Verification items for the finished model (mm, model axes). Face numbers are marked on the shaded views. Round coordinates to 2 decimals unless told otherwise and drop trailing zeros. Order: outer loops, then holes, each group sorted by start corner. A loop starts at its lowest first (then second) coordinate and runs counter-clockwise, first axis right, second up. Notation, with made-up numbers: M -38.5,0 L -29.5,0 A28 ccw -29.5,22 Z; hole C 5,88.25 d8. An arc over 180 degrees is marked long. Use one line per item in the form item = value. Start each with the question number.
Item 1: Cross-section at D-D on x = 14.5. Enter the section's corners in (y, z) (3 decimals).
Item 2: Cross-section at C-C on z = 0.8. Count the separate pieces of the cut face and the enclosed holes in it, then the cut area to 3 significant figures.
Item 3: Cross-section at B-B on x = -6. Enter the section's corners in (y, z) (3 decimals), then the cut area to 3 significant figures.
Item 4: Cross-section at A-A on y = -24.5. Enter the section's corners in (x, z) (3 decimals), then the cut area to 3 significant figures.
Item 5: Release check for a two-part mould opening along Z. For the marked faces 1 and 2 record: +Z half, -Z half, draft (parallel to the pull), parting line (faces both ways), or undercut.
Item 6: Go/stop test with flat-tipped pins: pin 1 Ø1.6 at (y, z) = (-81.5, 1.5) entering from +X; pin 2 Ø1.5 at (y, z) = (-7, 1.5) entering from +X; pin 3 Ø1.6 at (y, z) = (-74.5, 2) entering from -X. Record where each tip stops, or that it passes through.
Item 7: Thickness scan on probe 1 along Y at (x, z) = (-22, 1.2); probe 2 along Y at (x, z) = (-14.5, 0.75); probe 3 along X at (y, z) = (1, 1.5). Record the ranges inside material, lowest first. Write a range as [from, to].
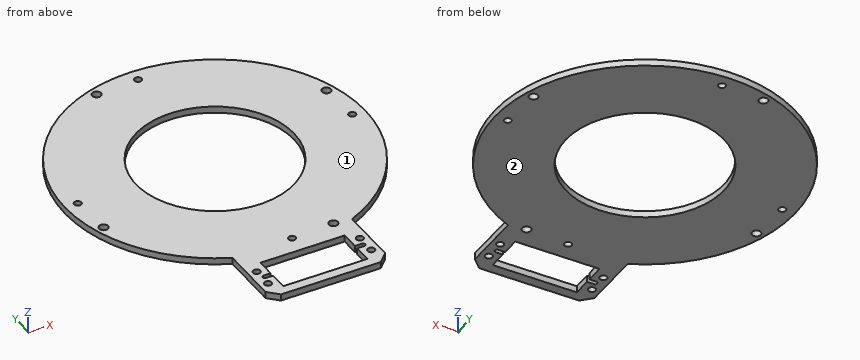
from build123d import *

# Parameters (mm, degrees)
F0_R     = 1.7272
F0_R_2   = 2.15265
F0_R_3   = 38.1
F1_DEPTH = 3.175
F2_SIZE  = 4.7625


# Not quite as in the source:
# - a feature names something its author has since deleted; it is built from what else it names


with BuildPart() as f1:
    # F0 (on Top) → F1 (new body)
    with BuildSketch(Plane.XY):
        with BuildLine():
            Line((28.86075, -99.6367724936), (28.86075, -66.3880200747))
            ThreePointArc((28.86075, -66.3880200747), (0, 72.39), (-28.86075, -66.3880200747))
            Line((-28.86075, -66.3880200747), (-28.86075, -99.6367724936))
            Line((-28.86075, -99.6367724936), (28.86075, -99.6367724936))
        make_face()
        with Locations((-24.892, -89.9847724936)):
            Circle(F0_R, mode=Mode.SUBTRACT)
        with Locations((-24.892, -80.2057724936)):
            Circle(F0_R, mode=Mode.SUBTRACT)
        with Locations((-65.2747423649, -20.5103744665)):
            Circle(F0_R_2, mode=Mode.SUBTRACT)
        with BuildLine():
            Line((-20.32, -94.8742724936), (-20.32, -86.1112724936))
            Line((-20.32, -86.1112724936), (-23.749, -86.1112724936))
            ThreePointArc((-23.749, -86.1112724936), (-24.765, -85.0952724936), (-23.749, -84.0792724936))
            Line((-23.749, -84.0792724936), (-20.32, -84.0792724936))
            Line((-20.32, -84.0792724936), (-20.32, -75.3162724936))
            Line((-20.32, -75.3162724936), (20.32, -75.3162724936))
            Line((20.32, -75.3162724936), (20.32, -84.0792724936))
            Line((20.32, -84.0792724936), (23.749, -84.0792724936))
            ThreePointArc((23.749, -84.0792724936), (24.765, -85.0952724936), (23.749, -86.1112724936))
            Line((23.749, -86.1112724936), (20.32, -86.1112724936))
            Line((20.32, -86.1112724936), (20.32, -94.8742724936))
            Line((20.32, -94.8742724936), (-20.32, -94.8742724936))
        make_face(mode=Mode.SUBTRACT)
        with Locations((24.892, -89.9847724936)):
            Circle(F0_R, mode=Mode.SUBTRACT)
        with Locations((24.892, -80.2057724936)):
            Circle(F0_R, mode=Mode.SUBTRACT)
        with Locations((0, -66.2293888929)):
            Circle(F0_R, mode=Mode.SUBTRACT)
        with Locations((20.5103744665, -65.2747423649)):
            Circle(F0_R_2, mode=Mode.SUBTRACT)
        with Locations((-66.2293888929, 0)):
            Circle(F0_R, mode=Mode.SUBTRACT)
        with Locations((-20.5103744665, 65.2747423649)):
            Circle(F0_R_2, mode=Mode.SUBTRACT)
        Circle(F0_R_3, mode=Mode.SUBTRACT)
        with Locations((66.2293888929, 0)):
            Circle(F0_R, mode=Mode.SUBTRACT)
        with Locations((65.2747423649, 20.5103744665)):
            Circle(F0_R_2, mode=Mode.SUBTRACT)
        with Locations((0, 66.2293888929)):
            Circle(F0_R, mode=Mode.SUBTRACT)
    extrude(amount=F1_DEPTH)

    # F2
    f2_edges = [f1.edges().sort_by_distance(p)[0] for p in [
        (-28.86075, -99.636772, 1.5875),
        (28.86075, -99.636772, 1.5875),
    ]]
    chamfer(f2_edges, length=F2_SIZE)


solid = f1.part
Output values:
q1.outline = M -99.637,0 L -94.874,0 L -94.874,3.175 L -99.637,3.175 Z; M -75.316,0 L -35.233,0 L -35.233,3.175 L -75.316,3.175 Z; M 35.233,0 L 70.923,0 L 70.923,3.175 L 35.233,3.175 Z
q2.separate_pieces = 1
q2.enclosed_holes = 14
q2.area = 12,600 mm2
q3.outline = M -99.637,0 L -94.874,0 L -94.874,3.175 L -99.637,3.175 Z; M -75.316,0 L -37.625,0 L -37.625,3.175 L -75.316,3.175 Z; M 37.625,0 L 72.141,0 L 72.141,3.175 L 37.625,3.175 Z
q3.area = 244 mm2
q4.outline = M -68.118,0 L -29.178,0 L -29.178,3.175 L -68.118,3.175 Z; M 29.178,0 L 68.118,0 L 68.118,3.175 L 29.178,3.175 Z
q4.area = 247 mm2
q5.face_1 = +Z half
q5.face_2 = -Z half
q6.pin_1 = 28.86
q6.pin_2 = 72.12
q6.pin_3 = -28.86
q7.probe_1 = [-99.64, -86.11], [-84.08, -31.11], [31.11, 63.72], [66.83, 68.97]
q7.probe_2 = [-99.64, -94.87], [-75.32, -35.23], [35.23, 70.92]
q7.probe_3 = [-72.38, -67.64], [-64.82, -38.09], [38.09, 64.82], [67.64, 72.38]
